```python
from build123d import *

# Parameters (mm, degrees)
F0_W         = 29.492739588
F0_H         = 29.492739588
F0_R         = 10.6622653611
F0_R_2       = 13.2
F0_R_3       = 11.2
F1_DEPTH     = 7
F2_T4_ANGLE  = 112.5181364767
F2_T10_ANGLE = 112.5181364767
F2_T16_ANGLE = 112.5181364767
F2_T22_ANGLE = 112.5181364767
F2_T28_ANGLE = 112.5181364767
F2_T34_ANGLE = 112.5181364767


# Not quite as in the source:
# - a fillet or chamfer that OpenCascade refuses, or shapes differently, is made with other operations: its cross-section is extruded or revolved along the edge and cut away or added


with BuildPart() as f1:
    # F0 (on Top) → F1 (new body)
    with BuildSketch(Plane.XY):
        with Locations((0, 36.7929209024)):
            Rectangle(F0_W, F0_H)
        with Locations((0, 36.7929209024)):
            Circle(F0_R, mode=Mode.SUBTRACT)
        with BuildLine():
            Line((14.746369794, 22.0465511084), (-14.746369794, 22.0465511084))
            ThreePointArc((-14.746369794, 22.0465511084), (-23.115726428, 13.3458708757), (-26.4660582227, 1.747455301))
            Line((-26.4660582227, 1.747455301), (-11.7196884287, -23.7940064094))
            ThreePointArc((-11.7196884287, -23.7940064094), (0, -26.6917417515), (11.7196884287, -23.7940064094))
            Line((11.7196884287, -23.7940064094), (26.4660582227, 1.747455301))
            ThreePointArc((26.4660582227, 1.747455301), (23.115726428, 13.3458708757), (14.746369794, 22.0465511084))
        make_face()
        Circle(F0_R_2, mode=Mode.SUBTRACT)
        Polygon((52.0075199331, -12.998914493), (26.4660582227, 1.747455301), (11.7196884287, -23.7940064094), (37.2611501391, -38.5403762034), align=None)
        with Locations((31.8636041809, -18.3964604512)):
            Circle(F0_R, mode=Mode.SUBTRACT)
        Polygon((-11.7196884287, -23.7940064094), (-26.4660582227, 1.747455301), (-52.0075199331, -12.998914493), (-37.2611501391, -38.5403762034), align=None)
        with Locations((-31.8636041809, -18.3964604512)):
            Circle(F0_R, mode=Mode.SUBTRACT)
        Circle(F0_R_2)
        Circle(F0_R_3, mode=Mode.SUBTRACT)
    extrude(amount=F1_DEPTH)

    # F2: fillet of radius 5 on 6 edges, made by hand


with BuildPart() as f2_tool2:
    # F2_s3 → F2_t4 (revolve)
    with BuildSketch(Plane(origin=(-1.2804779727, -0.0837234298, 0), x_dir=(0, 0, 1), z_dir=(0.9978692621, 0.0652451967, 0))):
        with BuildLine():
            ThreePointArc((2, -26.0057199962), (5.5355339059, -24.5412539021), (7, -21.0057199962))
            Line((7, -21.0057199962), (7, -26.0057199962))
            Line((7, -26.0057199962), (2, -26.0057199962))
        make_face()
    revolve(axis=Axis((-1.336401015, 0.7715714858, 7), (0, 0, 1)), revolution_arc=F2_T4_ANGLE)

    split(bisect_by=Plane.YZ.offset(-14.746369794), keep=Keep.BOTTOM)

    split(bisect_by=Plane(origin=(-7.373184897, 12.7707308552, 0), x_dir=(0, 0, 1), z_dir=(-0.5, 0.8660254038, 0)), keep=Keep.TOP)


with BuildPart() as f1_1:
    add(f1.part)

    # F2_t1: cut F2_tool2
    add(f2_tool2.part, mode=Mode.SUBTRACT)


with BuildPart() as f2_tool8:
    # F2_s9 → F2_t10 (revolve)
    with BuildSketch(Plane(origin=(0.5677323692, 1.1507881683, 0), x_dir=(0, 0, 1), z_dir=(-0.4424306333, -0.896802729, 0))):
        with BuildLine():
            ThreePointArc((2, -26.0057199962), (5.5355339059, -24.5412539021), (7, -21.0057199962))
            Line((7, -21.0057199962), (7, -26.0057199962))
            Line((7, -26.0057199962), (2, -26.0057199962))
        make_face()
    revolve(axis=Axis((1.336401015, 0.7715714858, 7), (0, 0, 1)), revolution_arc=F2_T10_ANGLE)

    split(bisect_by=Plane(origin=(7.373184897, 12.7707308552, 0), x_dir=(0, 0, 1), z_dir=(0.5, 0.8660254038, 0)), keep=Keep.TOP)

    split(bisect_by=Plane.YZ.offset(14.746369794), keep=Keep.TOP)


with BuildPart() as f1_2:
    add(f1_1.part)

    # F2_t7: cut F2_tool8
    add(f2_tool8.part, mode=Mode.SUBTRACT)


with BuildPart() as f2_tool14:
    # F2_s15 → F2_t16 (revolve)
    with BuildSketch(Plane(origin=(0.7127456035, -1.0670647384, 0), x_dir=(0, 0, 1), z_dir=(-0.5554386289, 0.8315575323, 0))):
        with BuildLine():
            ThreePointArc((2, -26.0057199962), (5.5355339059, -24.5412539021), (7, -21.0057199962))
            Line((7, -21.0057199962), (7, -26.0057199962))
            Line((7, -26.0057199962), (2, -26.0057199962))
        make_face()
    revolve(axis=Axis((0, -1.5431429715, 7), (0, 0, 1)), revolution_arc=F2_T16_ANGLE)

    split(bisect_by=Plane(origin=(7.373184897, -12.7707308552, 0), x_dir=(0, 0, 1), z_dir=(0.5, -0.8660254038, 0)), keep=Keep.TOP)

    split(bisect_by=Plane(origin=(-7.373184897, -12.7707308552, 0), x_dir=(0, 0, 1), z_dir=(-0.5, -0.8660254038, 0)), keep=Keep.TOP)


with BuildPart() as f1_3:
    add(f1_2.part)

    # F2_t13: cut F2_tool14
    add(f2_tool14.part, mode=Mode.SUBTRACT)


with BuildPart() as f2_tool20:
    # F2_s21 → F2_t22 (revolve)
    with BuildSketch(Plane(origin=(0.5677323692, 1.1507881683, 0), x_dir=(0, 0, 1), z_dir=(-0.4424306333, -0.896802729, 0))):
        with BuildLine():
            ThreePointArc((5, -26.0057199962), (1.4644660941, -24.5412539021), (0, -21.0057199962))
            Line((0, -21.0057199962), (0, -26.0057199962))
            Line((0, -26.0057199962), (5, -26.0057199962))
        make_face()
    revolve(axis=Axis((1.336401015, 0.7715714858, 0), (0, 0, 1)), revolution_arc=F2_T22_ANGLE)

    split(bisect_by=Plane(origin=(7.373184897, 12.7707308552, 0), x_dir=(0, 0, 1), z_dir=(0.5, 0.8660254038, 0)), keep=Keep.TOP)

    split(bisect_by=Plane.YZ.offset(14.746369794), keep=Keep.TOP)


with BuildPart() as f1_4:
    add(f1_3.part)

    # F2_t19: cut F2_tool20
    add(f2_tool20.part, mode=Mode.SUBTRACT)


with BuildPart() as f2_tool26:
    # F2_s27 → F2_t28 (revolve)
    with BuildSketch(Plane(origin=(0.7127456035, -1.0670647384, 0), x_dir=(0, 0, 1), z_dir=(-0.5554386289, 0.8315575323, 0))):
        with BuildLine():
            ThreePointArc((5, -26.0057199962), (1.4644660941, -24.5412539021), (0, -21.0057199962))
            Line((0, -21.0057199962), (0, -26.0057199962))
            Line((0, -26.0057199962), (5, -26.0057199962))
        make_face()
    revolve(axis=Axis((0, -1.5431429715, 0), (0, 0, 1)), revolution_arc=F2_T28_ANGLE)

    split(bisect_by=Plane(origin=(7.373184897, -12.7707308552, 0), x_dir=(0, 0, 1), z_dir=(0.5, -0.8660254038, 0)), keep=Keep.TOP)

    split(bisect_by=Plane(origin=(-7.373184897, -12.7707308552, 0), x_dir=(0, 0, 1), z_dir=(-0.5, -0.8660254038, 0)), keep=Keep.TOP)


with BuildPart() as f1_5:
    add(f1_4.part)

    # F2_t25: cut F2_tool26
    add(f2_tool26.part, mode=Mode.SUBTRACT)


with BuildPart() as f2_tool32:
    # F2_s33 → F2_t34 (revolve)
    with BuildSketch(Plane(origin=(-1.2804779727, -0.0837234298, 0), x_dir=(0, 0, 1), z_dir=(0.9978692621, 0.0652451967, 0))):
        with BuildLine():
            ThreePointArc((5, -26.0057199962), (1.4644660941, -24.5412539021), (0, -21.0057199962))
            Line((0, -21.0057199962), (0, -26.0057199962))
            Line((0, -26.0057199962), (5, -26.0057199962))
        make_face()
    revolve(axis=Axis((-1.336401015, 0.7715714858, 0), (0, 0, 1)), revolution_arc=F2_T34_ANGLE)

    split(bisect_by=Plane.YZ.offset(-14.746369794), keep=Keep.BOTTOM)

    split(bisect_by=Plane(origin=(-7.373184897, 12.7707308552, 0), x_dir=(0, 0, 1), z_dir=(-0.5, 0.8660254038, 0)), keep=Keep.TOP)


with BuildPart() as f1_6:
    add(f1_5.part)

    # F2_t31: cut F2_tool32
    add(f2_tool32.part, mode=Mode.SUBTRACT)


solid = f1_6.part
```
Here's how the part is built. I have some questions about the finished solid (model axes, mm). Coordinates: 2 decimals unless noted, no trailing zeros. Order: outer loops, then holes, each group sorted by start corner. A loop starts at its lowest first (then second) coordinate and runs counter-clockwise, first axis right, second up. Notation, with made-up numbers: (27, 69) - (42, 69) arc R19 ccw to (42, 102) - close; hole circle Ø1 at (26, 37). An arc over 180 degrees is marked (long way). One line per question, with ' | ' between items. Start each with the question number.
1. If we section it at C-C (x = 41): Write out the boundary of the cut face in (y, z), and give its area (3 significant figures).
2. If we section it at A-A (y = 40.5): Write out the boundary of the cut face in (x, z), and give its area (3 significant figures).
3. If we mould it in two halves opening along Y, with no side actions, what happens to faces 1 (the flat face through (14.746, 37, 3)), 2 (the cylindrical face through (-11.19, 0.49, 3.45)), 3 (the flat face through (44.53, -25.95, 3.45))? For each: released by +Y, released by -Y, zero draft, split by the parting line, or undercut.
4. If we section it at B-B (x = 0): Write out the boundary of the cut face in (y, z).
5. I'm going to push flat-ended pins straight in: pin 1 Ø1.5 at (y, z) = (26, 6) entering from +X; pin 2 Ø17 at (x, y) = (31.86, -18.4) entering from +Z; pin 3 Ø3 at (y, z) = (9, 1) entering from -X; pin 4 Ø1 at (y, z) = (34.5, 5.5) entering from -X. Where does each tip first touch, or does it pass through?
6. If we section it at D-D (z = 5.75): Write out the boundary of the cut face in (x, y), and give its area (3 significant figures).
7. Please list where these lines run through material, in increasing order: line 1 along Y through (x, z) = (0, 3.5); line 2 along X through (y, z) = (-17.5, 5); line 3 along Y through (x, z) = (7, 5.5). Write a range as [from, to].
Model answer:
1) outline: (-32.06, 0) - (-23.89, 0) - (-23.89, 7) - (-32.06, 7) - close; (-12.9, 0) - (-6.64, 0) - (-6.64, 7) - (-12.9, 7) - close | area: 101 mm²
2) outline: (-14.75, 0) - (-10, 0) - (-10, 7) - (-14.75, 7) - close; (10, 0) - (14.75, 0) - (14.75, 7) - (10, 7) - close | area: 66.5 mm²
3) face 1: zero draft | face 2: undercut | face 3: released by -Y
4) outline: (-26.46, 3.5) arc R5 ccw to (-21.69, 0) - (-11.2, 0) - (-11.2, 7) - (-21.69, 7) arc R5 ccw to start; (11.2, 0) - (26.13, 0) - (26.13, 7) - (11.2, 7) - close; (47.46, 0) - (51.54, 0) - (51.54, 7) - (47.46, 7) - close
5) pin 1: stops at x = 14.75 | pin 2: passes through | pin 3: stops at x = -24.52 | pin 4: stops at x = -14.75
6) outline: (-52.01, -13) - (-37.26, -38.54) - (-9.96, -22.78) arc R23.46 ccw to (9.96, -22.78) - (37.26, -38.54) - (52.01, -13) - (24.71, 2.76) arc R23.46 ccw to (14.75, 20.02) - (14.75, 51.54) - (-14.75, 51.54) - (-14.75, 20.02) arc R23.46 ccw to (-24.71, 2.76) - close; hole circle Ø21.32 at (-31.86, -18.4); hole circle Ø22.4 at (0, 0); hole circle Ø21.32 at (0, 36.79); hole circle Ø21.32 at (31.86, -18.4) | area: 2,980 mm²
7) line 1: y = [-26.46, -11.2], [11.2, 26.13], [47.46, 51.54] | line 2: x = [-49.41, -42.49], [-21.24, 21.24], [42.49, 49.41] | line 3: y = [-24.21, -8.74], [8.74, 28.75], [44.84, 51.54]
